```python
from build123d import *

# Parameters (mm, degrees)
SKETCH1_W           = 31
SKETCH1_H           = 7
BOSS_EXTRUDE1_DEPTH = 5
SKETCH2_R           = 4.5
BOSS_EXTRUDE2_DEPTH = 5
SKETCH3_R           = 1.65
CUT_EXTRUDE1_DEPTH  = 37.732138517
SKETCH4_R           = 3.1
CUT_EXTRUDE2_DEPTH  = 2
FILLET1_R           = 0.5


with BuildPart() as part:
    # Sketch1 → Boss-Extrude1 (new body)
    with BuildSketch(Plane(origin=(0, 0, 0), x_dir=(1, 0, 0), z_dir=(0, 1, 0))):
        with Locations((15.5, 3.5)):
            Rectangle(SKETCH1_W, SKETCH1_H)
    extrude(amount=BOSS_EXTRUDE1_DEPTH)

    # Sketch2 → Boss-Extrude2 (add)
    with BuildSketch(Plane(origin=(0, 5, 0), x_dir=(1, 0, 0), z_dir=(0, 1, 0))):
        with Locations((31, 3.5)):
            Circle(SKETCH2_R)
        with Locations((0, 3.5)):
            Circle(SKETCH2_R)
    extrude(amount=-BOSS_EXTRUDE2_DEPTH)

    # Sketch3 → Cut-Extrude1 (cut, through all)
    with BuildSketch(Plane(origin=(0, 5, 0), x_dir=(1, 0, 0), z_dir=(0, 1, 0))):
        with Locations(Location((0, 3.5, 0), (0, 0, 270))):
            Circle(SKETCH3_R)
        with Locations(Location((31, 3.5, 0), (0, 0, 270))):
            Circle(SKETCH3_R)
    extrude(amount=-CUT_EXTRUDE1_DEPTH, mode=Mode.SUBTRACT)

    # Sketch4 → Cut-Extrude2 (cut)
    with BuildSketch(Plane(origin=(0, 5, 0), x_dir=(1, 0, 0), z_dir=(0, 1, 0))):
        with Locations(Location((0, 3.5, 0), (0, 0, 270))):
            Circle(SKETCH4_R)
        with Locations(Location((31, 3.5, 0), (0, 0, 270))):
            Circle(SKETCH4_R)
    extrude(amount=-CUT_EXTRUDE2_DEPTH, mode=Mode.SUBTRACT)

    # Fillet1
    fillet1_edges = [part.edges().sort_by_distance(p)[0] for p in [
        (15.5, 0, -7),
        (35.5, 0, -3.5),
        (15.5, 0, 0),
        (-4.5, 0, -3.5),
    ]]
    fillet(fillet1_edges, radius=FILLET1_R)


solid = part.part
```
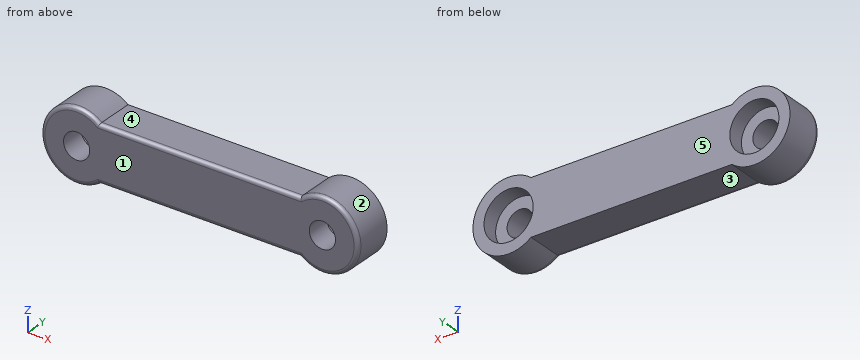
Model file for the job. Use its own axes, mm. Face numbers are marked on the shaded views. A direction names the side the tool comes from. Round coordinates to 2 decimals unless told otherwise and drop trailing zeros. Order: outer loops, then holes, each group sorted by start corner. A loop starts at its lowest first (then second) coordinate and runs counter-clockwise, first axis right, second up. Notation, with made-up numbers: (8, 19) -> (50, 19) arc R9 cw to (50, 31) -> close; hole circle Ø10 at (82.25, 61). An arc over 180 degrees is marked (long way). Use one line per item in the form item = value.
Item 1: Cut at A-A, the plane x = 0. Write the cut outline in (y, z), and give its area (3 significant figures).
Returned:
outline = (0, -7.5) arc R0.5 ccw to (0.5, -8) -> (5, -8) -> (5, -6.6) -> (3, -6.6) -> (3, -5.15) -> (0, -5.15) -> close; (0, -1.85) -> (3, -1.85) -> (3, -0.4) -> (5, -0.4) -> (5, 1) -> (0.5, 1) arc R0.5 ccw to (0, 0.5) -> close
area = 22.6 mm^2
Item 2: Flat gauge pins, fed straight in: pin 1 Ø3 at (y, z) = (3.5, -0.5) entering from -X; pin 2 Ø1.5 at (x, y) = (1.5, 1.5) entering from +Z; pin 3 Ø5 at (x, z) = (31.5, -3.5) entering from +Y. Where does each tip first touch, or does it go through?
Returned:
pin_1 = -4.24
pin_2 = 0.94
pin_3 = 3
Item 3: Tool access for the marked faces 3, 4 and 5: list every direction of +Z, -Z, +X, -X, +Y, -Y with a clear straight run to the whole face (end or side of a thin tool).
Returned:
face_3 = -Z, +Y, -Y
face_4 = +Z, +Y, -Y
face_5 = +Z, -Z, +X, -X, +Y
Item 4: Drill centre lines: line 1 (X direction, y = 0.7, z = -3.5); line 2 (X direction, y = 4.3, z = -3.5); line 3 (Z direction, x = 16, y = 2.25). Where is each one in solid material? Low to high.
Returned:
line_1 = -4.5 to -1.65, 1.65 to 29.35, 32.65 to 35.5
line_2 = -4.5 to -3.1, 3.1 to 27.9, 34.1 to 35.5
line_3 = -7 to 0
Item 5: Cut at D-D, the plane x = 12. Write the cut outline in (y, z), and give its area (3 significant figures).
Returned:
outline = (0, -6.5) arc R0.5 ccw to (0.5, -7) -> (5, -7) -> (5, 0) -> (0.5, 0) arc R0.5 ccw to (0, -0.5) -> close
area = 34.9 mm^2
Item 6: Cut at C-C, the plane y = 2.15. Write the cut outline in (x, z).
Returned:
outline = (2.83, -7) -> (28.17, -7) arc R4.5 ccw (long way) to (28.17, 0) -> (2.83, 0) arc R4.5 ccw (long way) to start; hole circle Ø3.3 at (0, -3.5); hole circle Ø3.3 at (31, -3.5)
Item 7: Pull direction X, two halves, no side cores. Call the marked faces 1 and 2: released by +X, released by -X, zero draft, split by the parting line, or undercut.
Returned:
face_1 = zero draft
face_2 = undercut
Item 8: Cut at B-B, the plane z = -3.5. Write the cut outline in (x, y), and give its area (3 significant figures).
Returned:
outline = (-4.5, 0.5) arc R0.5 ccw to (-4, 0) -> (-1.65, 0) -> (-1.65, 3) -> (-3.1, 3) -> (-3.1, 5) -> (-4.5, 5) -> close; (1.65, 0) -> (29.35, 0) -> (29.35, 3) -> (27.9, 3) -> (27.9, 5) -> (3.1, 5) -> (3.1, 3) -> (1.65, 3) -> close; (32.65, 0) -> (35, 0) arc R0.5 ccw to (35.5, 0.5) -> (35.5, 5) -> (34.1, 5) -> (34.1, 3) -> (32.65, 3) -> close
area = 155 mm^2
